Can you work these out from the model? Positions are in its coordinate system, mm. Face numbers are marked on the shaded views. Give positions to 0.01 mm unless a question says otherwise; leave off trailing zeros. Order: outer loops, then holes, each group sorted by start corner. A loop starts at its lowest first (then second) coordinate and runs counter-clockwise, first axis right, second up. Notation, with made-up numbers: (38.5, 54) - (62.5, 54) arc R29 ccw to (62.5, 81) - close; hole circle Ø9 at (-28.5, -10.75). An arc over 180 degrees is marked (long way). Return JSON: item names as keys, results as strings.
```python
from build123d import *

# Parameters (mm, degrees)
F0_R = 50
F2_R = 30
F4_T = -5
F5_R = 2.49999
F6_R = 7.5


# Not quite as in the source:
# - a fillet or chamfer is up to 0.001 mm smaller than in the source, because OpenCascade refuses the exact size


with BuildPart() as f3:
    # F0 (on Top) → F3 section 0
    with BuildSketch(Plane.XY):
        Circle(F0_R)
    # F2 (on offset) → F3 section 1
    with BuildSketch(Plane.XY.offset(100)):
        Circle(F2_R)
    loft()

    # F4
    f4_openings = [f3.faces().sort_by_distance(p)[0] for p in [
        (0, 0, 100),
    ]]
    offset(amount=F4_T, openings=f4_openings, kind=Kind.INTERSECTION)

    # F5 (radius 2.5 in the source; OpenCascade refuses exactly that, so slightly less here)
    f5_edges = [f3.edges().sort_by_distance(p)[0] for p in [
        (-30, 0, 100),
        (-24.90098, 0, 100),
    ]]
    fillet(f5_edges, radius=F5_R)

    # F6
    f6_edges = [f3.edges().sort_by_distance(p)[0] for p in [
        (-50, 0, 0),
        (-43.90098, 0, 5),
    ]]
    fillet(f6_edges, radius=F6_R)


solid = f3.part
```
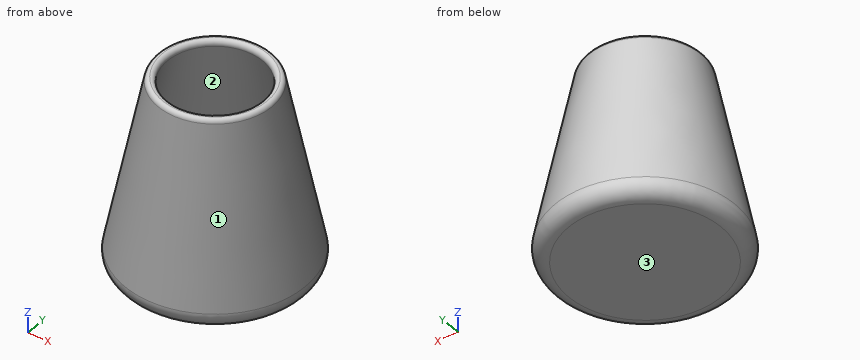
1. For pin 1 Ø4 at (y, z) = (12.5, 68) entering from -X; pin 2 Ø10 at (x, z) = (33, 19.5) entering from +Y; pin 3 Ø6 at (y, z) = (-21, 47) entering from -X, each with a flat end and sliding along its axis, tell me the tip position at first contact or that it passes through.
Checks:
{"pin 1": "x = -34.98", "pin 2": "y = 36.82", "pin 3": "x = -36.54"}
2. Thinking about a two-plate mould opening in Z: for the marked faces 1, 2 and 3, which applies, +Z half, -Z half, draft (parallel to the pull), parting line (faces both ways), or undercut?
Checks:
{"face 1": "+Z half", "face 2": "undercut", "face 3": "-Z half"}
3. If I drill on L1, parallel to Z at x = -18, y = 12.5; L2, parallel to X at y = 24.5, z = 25; L3, parallel to Y at x = -30, z = 21.5, over which ranges is the centre line in solid material (lowest first)? Write a range as [from, to].
Checks:
{"L1": "[0, 5]", "L2": "[-37.75, -31.49], [31.49, 37.75]", "L3": "[-34.47, -27.36], [27.36, 34.47]"}
4. Suppose I cut it at C-C (z = 90). List the corners of the cut face in (x, y) for me, plus the area to 3 significant figures.
Checks:
{"outline": "circle Ø64 at (0, 0); hole circle Ø53.8 at (0, 0)", "area": "944 mm^2"}
5. Suppose I cut it at B-B (z = 12). List the corners of the cut face in (x, y) for me.
Checks:
{"outline": "circle Ø95.2 at (0, 0); hole circle Ø84.47 at (0, 0)"}
